from build123d import *

# Parameters (mm, degrees)
SKETCH1_W                      = 99
SKETCH1_H                      = 100
BOSS_EXTRUDE1_DEPTH            = 1.5875
CUT_EXTRUDE1_DEPTH             = 71.375920287
CUT_EXTRUDE2_DEPTH             = 71.375920287
CUT_EXTRUDE3_DEPTH             = 71.375920287
CUT_EXTRUDE4_DEPTH             = 71.375920287
CUT_EXTRUDE5_DEPTH             = 71.375920287
CUT_EXTRUDE6_DEPTH             = 71.375920287
CUT_EXTRUDE7_DEPTH             = 71.375920287
CUT_EXTRUDE8_DEPTH             = 71.375920287
SKETCH10_W                     = 50
SKETCH10_H                     = 16.6
BOSS_EXTRUDE2_DEPTH            = 0.1
SKETCH11_W                     = 50
SKETCH11_H                     = 16.6
BOSS_EXTRUDE3_DEPTH            = 0.1
SKETCH12_W                     = 50
SKETCH12_H                     = 16.6
BOSS_EXTRUDE4_DEPTH            = 0.1
SKETCH13_W                     = 50
SKETCH13_H                     = 16.6
BOSS_EXTRUDE5_DEPTH            = 0.1
SKETCH14_W                     = 50
SKETCH14_H                     = 16.6
BOSS_EXTRUDE6_DEPTH            = 0.1
SKETCH15_W                     = 55
SKETCH15_H                     = 5
BOSS_EXTRUDE7_DEPTH            = 0.1
SKETCH16_W                     = 4.9
SKETCH16_H                     = 5
BOSS_EXTRUDE8_DEPTH            = 0.1
F_000_CLEARANCE_HOLE1_D        = 1
F_000_CLEARANCE_HOLE2_D        = 1
F_000_CLEARANCE_HOLE2_DEPTH    = 1.6875
F_50_0_07_DIAMETER_HOLE1_D     = 1.778
F_50_0_07_DIAMETER_HOLE1_DEPTH = 1.6875
F_50_0_07_DIAMETER_HOLE2_D     = 1.778


with BuildPart() as part:
    # Sketch1 → Boss-Extrude1 (new body)
    with BuildSketch(Plane.XY.offset(1.5875)):
        Rectangle(SKETCH1_W, SKETCH1_H)
    extrude(amount=-BOSS_EXTRUDE1_DEPTH)

    # Sketch2 → Cut-Extrude1 (cut, through all)
    with BuildSketch(Plane(origin=(0, 0, 0), x_dir=(-1, 0, 0), z_dir=(0, 0, -1))):
        with BuildLine():
            Line((48, -42.481934729), (48, -50))
            Line((48, -50), (49.5, -50))
            Line((49.5, -50), (49.5, -40.164608684))
            ThreePointArc((49.5, -40.164608684), (48.40772422, -41.101717355), (48, -42.481934729))
        make_face()
    extrude(amount=-CUT_EXTRUDE1_DEPTH, mode=Mode.SUBTRACT)

    # Sketch3 → Cut-Extrude2 (cut, through all)
    with BuildSketch(Plane(origin=(0, 0, 0), x_dir=(-1, 0, 0), z_dir=(0, 0, -1))):
        with BuildLine():
            Line((48, -48), (42.481934729, -48))
            ThreePointArc((42.481934729, -48), (40.888196984, -48.562223471), (40, -50))
            Line((40, -50), (48, -50))
            Line((48, -50), (48, -48))
        make_face()
    extrude(amount=-CUT_EXTRUDE2_DEPTH, mode=Mode.SUBTRACT)

    # Sketch4 → Cut-Extrude3 (cut, through all)
    with BuildSketch(Plane(origin=(0, 0, 0), x_dir=(-1, 0, 0), z_dir=(0, 0, -1))):
        with BuildLine():
            Line((-42.481934729, -48), (-49.5, -48))
            Line((-49.5, -48), (-49.5, -50))
            Line((-49.5, -50), (-40, -50))
            ThreePointArc((-40, -50), (-40.888196984, -48.562223471), (-42.481934729, -48))
        make_face()
    extrude(amount=-CUT_EXTRUDE3_DEPTH, mode=Mode.SUBTRACT)

    # Sketch5 → Cut-Extrude4 (cut, through all)
    with BuildSketch(Plane(origin=(0, 0, 0), x_dir=(-1, 0, 0), z_dir=(0, 0, -1))):
        with BuildLine():
            Line((-48, -48), (-48, -42.481934729))
            ThreePointArc((-48, -42.481934729), (-48.40772422, -41.101717355), (-49.5, -40.164608684))
            Line((-49.5, -40.164608684), (-49.5, -48))
            Line((-49.5, -48), (-48, -48))
        make_face()
    extrude(amount=-CUT_EXTRUDE4_DEPTH, mode=Mode.SUBTRACT)

    # Sketch6 → Cut-Extrude5 (cut, through all)
    with BuildSketch(Plane(origin=(0, 0, 0), x_dir=(-1, 0, 0), z_dir=(0, 0, -1))):
        with BuildLine():
            Line((-48, 42.481934729), (-48, 50))
            Line((-48, 50), (-49.5, 50))
            Line((-49.5, 50), (-49.5, 40.164608684))
            ThreePointArc((-49.5, 40.164608684), (-48.40772422, 41.101717355), (-48, 42.481934729))
        make_face()
    extrude(amount=-CUT_EXTRUDE5_DEPTH, mode=Mode.SUBTRACT)

    # Sketch7 → Cut-Extrude6 (cut, through all)
    with BuildSketch(Plane(origin=(0, 0, 0), x_dir=(-1, 0, 0), z_dir=(0, 0, -1))):
        with BuildLine():
            Line((-48, 48), (-42.481934729, 48))
            ThreePointArc((-42.481934729, 48), (-40.888196984, 48.562223471), (-40, 50))
            Line((-40, 50), (-48, 50))
            Line((-48, 50), (-48, 48))
        make_face()
    extrude(amount=-CUT_EXTRUDE6_DEPTH, mode=Mode.SUBTRACT)

    # Sketch8 → Cut-Extrude7 (cut, through all)
    with BuildSketch(Plane(origin=(0, 0, 0), x_dir=(-1, 0, 0), z_dir=(0, 0, -1))):
        with BuildLine():
            Line((42.481934729, 48), (49.5, 48))
            Line((49.5, 48), (49.5, 50))
            Line((49.5, 50), (40, 50))
            ThreePointArc((40, 50), (40.888196984, 48.562223471), (42.481934729, 48))
        make_face()
    extrude(amount=-CUT_EXTRUDE7_DEPTH, mode=Mode.SUBTRACT)

    # Sketch9 → Cut-Extrude8 (cut, through all)
    with BuildSketch(Plane(origin=(0, 0, 0), x_dir=(-1, 0, 0), z_dir=(0, 0, -1))):
        with BuildLine():
            Line((48, 48), (48, 42.481934729))
            ThreePointArc((48, 42.481934729), (48.40772422, 41.101717355), (49.5, 40.164608684))
            Line((49.5, 40.164608684), (49.5, 48))
            Line((49.5, 48), (48, 48))
        make_face()
    extrude(amount=-CUT_EXTRUDE8_DEPTH, mode=Mode.SUBTRACT)

    # Sketch10 → Boss-Extrude2 (add)
    with BuildSketch(Plane.XY.offset(1.5875)):
        with Locations((0, 31.7)):
            Rectangle(SKETCH10_W, SKETCH10_H)
    extrude(amount=BOSS_EXTRUDE2_DEPTH)

    # Sketch11 → Boss-Extrude3 (add)
    with BuildSketch(Plane.XY.offset(1.5875)):
        with Locations((0, 14.6)):
            Rectangle(SKETCH11_W, SKETCH11_H)
    extrude(amount=BOSS_EXTRUDE3_DEPTH)

    # Sketch12 → Boss-Extrude4 (add)
    with BuildSketch(Plane.XY.offset(1.5875)):
        with Locations((0, -2.5)):
            Rectangle(SKETCH12_W, SKETCH12_H)
    extrude(amount=BOSS_EXTRUDE4_DEPTH)

    # Sketch13 → Boss-Extrude5 (add)
    with BuildSketch(Plane.XY.offset(1.5875)):
        with Locations((0, -19.6)):
            Rectangle(SKETCH13_W, SKETCH13_H)
    extrude(amount=BOSS_EXTRUDE5_DEPTH)

    # Sketch14 → Boss-Extrude6 (add)
    with BuildSketch(Plane.XY.offset(1.5875)):
        with Locations((0, -36.7)):
            Rectangle(SKETCH14_W, SKETCH14_H)
    extrude(amount=BOSS_EXTRUDE6_DEPTH)

    # Sketch15 → Boss-Extrude7 (add)
    with BuildSketch(Plane.XY.offset(1.5875)):
        with Locations((2.5, 42.6)):
            Rectangle(SKETCH15_W, SKETCH15_H)
    extrude(amount=BOSS_EXTRUDE7_DEPTH)

    # Sketch16 → Boss-Extrude8 (add)
    with BuildSketch(Plane.XY.offset(1.5875)):
        with Locations((27.55, -42.5)):
            Rectangle(SKETCH16_W, SKETCH16_H)
    extrude(amount=BOSS_EXTRUDE8_DEPTH)

    # #000 Clearance Hole1 (through all)
    with Locations(Plane.XY.offset(1.5875)):
        with Locations((41.5, -35)):
            Hole(F_000_CLEARANCE_HOLE1_D / 2)

    # #000 Clearance Hole2
    with Locations(Plane(origin=(0, 0, 0), x_dir=(-1, 0, 0), z_dir=(0, 0, -1))):
        with Locations((-35, 41.5), (35, -41.5), (41.5, 35)):
            Hole(F_000_CLEARANCE_HOLE2_D / 2, depth=F_000_CLEARANCE_HOLE2_DEPTH)

    # #50 (0.07) Diameter Hole1
    with Locations(Plane(origin=(0, 0, 0), x_dir=(-1, 0, 0), z_dir=(0, 0, -1))):
        with Locations((-35, 35), (-43.5, -37.5), (-35, -35), (37.5, -43.5), (35, -35), (43.5, 37.5), (35, 35)):
            Hole(F_50_0_07_DIAMETER_HOLE1_D / 2, depth=F_50_0_07_DIAMETER_HOLE1_DEPTH)

    # #50 (0.07) Diameter Hole2 (through all)
    with Locations(Plane.XY.offset(1.5875)):
        with Locations((37.5, 43.5)):
            Hole(F_50_0_07_DIAMETER_HOLE2_D / 2)


solid = part.part
Can you work these out from the model? Positions are in its coordinate system, mm. Give positions to 0.01 mm unless a question says otherwise; leave off trailing zeros. Loops run counter-clockwise (first coordinate to the right, second up) from the corner with the lowest first, then second, coordinate; pieces in that order, holes last. Notation, with made-up numbers: (57, -17.75) -> (76, -17.75) arc R11 ccw to (76, -10.75) -> close; hole circle Ø3 at (-27.5, 30.5). An arc over 180 degrees is marked (long way). Return JSON: item names as keys, results as strings.
Q1. For pin 1 Ø1 at (x, y) = (-35.5, -30.5) entering from +Z; pin 2 Ø1.1 at (x, y) = (37.5, 43.5) entering from +Z; pin 3 Ø0.8 at (y, z) = (-45.5, 1) entering from +X; pin 4 Ø0.5 at (x, z) = (-45, 1) entering from +Y, each with a flat end and sliding along its axis, tell me the tip position at first contact or that it passes through.
Checks:
{"pin 1": "stops at z = 1.59", "pin 2": "passes through", "pin 3": "stops at x = 48", "pin 4": "stops at y = 48"}
Q2. I need wall thicknesses on probe 1 along Y at (x, z) = (35, 0.4); probe 2 along Y at (x, z) = (-35, 0.5); probe 3 along X at (y, z) = (-35, 0.85). Which ranges of each line are inside material? Lowest first, please.
Checks:
{"probe 1": "y = -50 to -35.89, -34.11 to 34.11, 35.89 to 41, 42 to 50", "probe 2": "y = -50 to -42, -41 to -35.89, -34.11 to 34.11, 35.89 to 50", "probe 3": "x = -49.5 to -35.89, -34.11 to 34.11, 35.89 to 41, 42 to 49.5"}
Q3. I want a section at A-A, the plane x = 27. List the corners of the cut face in (y, z) for me, then the cut area to 3 significant figures.
Checks:
{"outline": "(-50, 0) -> (50, 0) -> (50, 1.59) -> (45.1, 1.59) -> (45.1, 1.69) -> (40.1, 1.69) -> (40.1, 1.59) -> (-40, 1.59) -> (-40, 1.69) -> (-45, 1.69) -> (-45, 1.59) -> (-50, 1.59) -> close", "area": "160 mm2"}
